Design review of the part built by this model. Coordinates are the model's own, in mm. A direction names the side the tool comes from. Coordinates: 2 decimals unless noted, no trailing zeros. Loops run counter-clockwise (first coordinate to the right, second up) from the corner with the lowest first, then second, coordinate; pieces in that order, holes last. Notation, with made-up numbers: (11.25, 21) - (62.25, 21) arc R32 ccw to (62.25, 57) - close; hole circle Ø2 at (75, 54). An arc over 180 degrees is marked (long way). Use one line per item in the form item = value. Start each with the question number.
(1) Add section A-A (z = -9.5). State the section outline as (x, y) points.
(2) The part is to be moulded in two halves that separate along Y. For faces 1 (the face through (493, 36, -16)), 2 (the face through (0, 19.1, 0.4)), 3 (the face through (493, -4, -14)), 4 (the face through (507, 32, -18)), say which applies: pulls with the +Y half, pulls with the -Y half, needs draft (parallel to the pull), parting line crosses it, or undercut.
(3) Clearance check with flat-ended pins moving along their axes: pin 1 Ø24 at (x, y) = (649.5, 11) entering from -Z; pin 2 Ø4 at (x, y) = (654.5, 8.5) entering from -Z. State where each tip first meets the part, or that it passes through.
(4) Add section C-C (y = 24.5). State the section outline as (x, z) points.
(5) Tool access review of faces 5 (the face through (493, 16, 0)), 6 (the face through (493, 16, 4)): name each direction out of +Z, -Z, +X, -X, +Y, -Y from which nothing blocks a thin tool from reaching the whole face with its end or side.
(6) For L1, parallel to Y at x = 242, z = -10; L2, parallel to Z at x = 484, y = 13.5; L3, parallel to Y at x = 811, z = -32, list the stretches that pass through material, from the lowest coordinate up.
(7) Add section B-B (x = 287.5). State the section outline as (y, z) points, plus the area to 3 significant figures.
```python
from build123d import *

# Parameters (mm, degrees)
EXTRUDE_1_DEPTH     = 1000
SKETCH_2_W          = 8.555369223
SKETCH_2_H          = 36.536948801
CUT_EXTRUDE_1_DEPTH = 1001


with BuildPart() as part:
    # Эскиз1 → Вытянуть-Тонкостенный1 (new body)
    with BuildSketch(Plane(origin=(0, 0, 0), x_dir=(0, 0, -1), z_dir=(1, 0, 0))):
        with BuildLine():
            Line((-4, 31), (-4, 1))
            ThreePointArc((-4, 1), (-2.535533906, -2.535533906), (1, -4))
            Line((1, -4), (31, -4))
            ThreePointArc((31, -4), (34.535533906, -2.535533906), (36, 1))
            Line((36, 1), (36, 31))
            ThreePointArc((36, 31), (34.535533906, 34.535533906), (31, 36))
            Line((31, 36), (1, 36))
            ThreePointArc((1, 36), (-2.535533906, 34.535533906), (-4, 31))
        make_face()
        with BuildLine():
            Line((0, 31), (0, 1))
            ThreePointArc((0, 1), (0.292893219, 0.292893219), (1, 0))
            Line((1, 0), (31, 0))
            ThreePointArc((31, 0), (31.707106781, 0.292893219), (32, 1))
            Line((32, 1), (32, 31))
            ThreePointArc((32, 31), (31.707106781, 31.707106781), (31, 32))
            Line((31, 32), (1, 32))
            ThreePointArc((1, 32), (0.292893219, 31.707106781), (0, 31))
        make_face(mode=Mode.SUBTRACT)
    extrude(amount=EXTRUDE_1_DEPTH)

    # Эскиз2 → Вырез-Вытянуть1 (cut, through all)
    with BuildSketch(Plane(origin=(1000, 0, 0), x_dir=(0, 0, -1), z_dir=(1, 0, 0))):
        with Locations((32.277684611, 13.731525599)):
            Rectangle(SKETCH_2_W, SKETCH_2_H)
    extrude(amount=-CUT_EXTRUDE_1_DEPTH, mode=Mode.SUBTRACT)


solid = part.part
```
Computed values:
q1.outline = (0, -4) - (1000, -4) - (1000, 0) - (0, 0) - close; (0, 32) - (1000, 32) - (1000, 36) - (0, 36) - close
q2.face_1 = pulls with the +Y half
q2.face_2 = needs draft
q2.face_3 = pulls with the -Y half
q2.face_4 = undercut
q3.pin_1 = -28
q3.pin_2 = 0
q4.outline = (0, 0) - (1000, 0) - (1000, 4) - (0, 4) - close
q5.face_5 = -Z, +X, -X
q5.face_6 = +Z, +X, -X, +Y, -Y
q6.L1 = -4 to 0, 32 to 36
q6.L2 = 0 to 4
q6.L3 = 32 to 35.9
q7.outline = (-4, -28) - (0, -28) - (0, -1) arc R1 cw to (1, 0) - (31, 0) arc R1 cw to (32, -1) - (32, -35.9) arc R5 ccw to (36, -31) - (36, -1) arc R5 ccw to (31, 4) - (1, 4) arc R5 ccw to (-4, -1) - close
q7.area = 400 mm^2
